Model file for the job. Use its own axes, mm. Face numbers are marked on the shaded views. A direction names the side the tool comes from. Give positions to 0.01 mm unless a question says otherwise; leave off trailing zeros. Loops run counter-clockwise (first coordinate to the right, second up) from the corner with the lowest first, then second, coordinate; pieces in that order, holes last. Notation, with made-up numbers: (-24.5, 34.25) - (-16.5, 34.25) arc R18 ccw to (-16.5, 46.25) - close; hole circle Ø8 at (-15, 10.5). An arc over 180 degrees is marked (long way). Answer as CSV lines item,"result". Start each with the question number.
Item 1: Saw through at C-C on y = 1.75. Give the cut face in (x, z).
Item 2: Drill centre lines: L1, parallel to X at y = 5.5, z = 0; L2, parallel to Y at x = 5, z = 0; L3, parallel to X at y = 1.25, z = 1. Where is each one in solid material? Low to high. Write a range as from..to.
Item 3: Tool access for the marked faces 4 and 5: list every direction of +Z, -Z, +X, -X, +Y, -Y with a clear straight run to the whole face (end or side of a thin tool).
Item 4: Pull direction X, two halves, no side cores. Call the marked faces 1, 2 and 3: pulls with the +X half, pulls with the -X half, needs draft (parallel to the pull), parting line crosses it, or undercut.
Item 5: Pin check, flat tips, straight feed: pin 1 (3 mm diameter, centred on x = 0.5, y = 7, fed in from -Z); pin 2 (1 mm diameter, centred on x = -1.5, y = 3, fed in from +Z); pin 3 (2 mm diameter, centred on x = -1.5, y = 0.5, fed in from +Z). Stop position of each tip, or through.
from build123d import *

# Parameters (mm, degrees)
SKETCH_1_R           = 6
SKETCH_1_R_2         = 1.5
EXTRUDE_1_DEPTH      = 0.9
EXTRUDE_2_DEPTH      = 7.3
EXTRUDE_2_DEPTH_BACK = 1.3
SKETCH_2_R           = 2.45
SKETCH_2_R_2         = 1.5
SKETCH_3_OUTSIDE_W   = 17.806
SKETCH_3_OUTSIDE_H   = 17.806
SKETCH_3_OUTSIDE_R   = 2.425
SKETCH_3_OUTSIDE_R_2 = 1.5
CUT_EXTRUDE_1_DEPTH  = 2
FILLET_1_R           = 0.1
FILLET_2_R           = 0.1
CHAMFER_1_SIZE       = 0.4
CHAMFER_1_SIZE2      = 1


with BuildPart() as part:
    # 草图1 → 凸台-拉伸1 (new body)
    with BuildSketch(Plane(origin=(0, 0, 0), x_dir=(1, 0, 0), z_dir=(0, 1, 0))):
        with Locations(Location((0, 0, 0), (0, 0, 270))):
            Circle(SKETCH_1_R)
        with Locations(Location((0, 0, 0), (0, 0, 270))):
            Circle(SKETCH_1_R_2, mode=Mode.SUBTRACT)
    extrude(amount=EXTRUDE_1_DEPTH)

    # 草图2 → 凸台-拉伸2 (add, two sides: drawn at the far end of the back side and taken through both)
    with BuildSketch(Plane(origin=(0, 0.9, 0), x_dir=(1, 0, 0), z_dir=(0, 1, 0)).offset(-EXTRUDE_2_DEPTH_BACK)):
        with Locations(Location((0, 0, 0), (0, 0, 270))):
            Circle(SKETCH_2_R)
        with Locations(Location((0, 0, 0), (0, 0, 270))):
            Circle(SKETCH_2_R_2, mode=Mode.SUBTRACT)
    extrude(amount=EXTRUDE_2_DEPTH + EXTRUDE_2_DEPTH_BACK)

    # 草图3 outside → 切除-拉伸1 (cut)
    # profile 1 of 2: a face of its own
    with BuildSketch(Plane(origin=(0, 8.2, 0), x_dir=(1, 0, 0), z_dir=(0, 1, 0))):
        Rectangle(SKETCH_3_OUTSIDE_W, SKETCH_3_OUTSIDE_H)
        with Locations(Location((0, 0, 0), (0, 0, 270))):
            Circle(SKETCH_3_OUTSIDE_R, mode=Mode.SUBTRACT)
    # profile 2 of 2: a face of its own
    with BuildSketch(Plane(origin=(0, 8.2, 0), x_dir=(1, 0, 0), z_dir=(0, 1, 0))):
        with Locations(Location((0, 0, 0), (0, 0, 270))):
            Circle(SKETCH_3_OUTSIDE_R_2)
    extrude(amount=-CUT_EXTRUDE_1_DEPTH, mode=Mode.SUBTRACT)

    # 圆角1
    fillet_1_edges = [part.edges().sort_by_distance(p)[0] for p in [
        (0, -0.4, -2.45),
        (0, -0.4, -1.5),
        (0, 8.2, -1.5),
        (0, 8.2, -2.425),
    ]]
    fillet(fillet_1_edges, radius=FILLET_1_R)

    # 圆角2
    # the kernel refuses this fillet: 0.1 mm, written as the material it takes off along each edge
    with BuildSketch(Plane(origin=(0, 6.2, 0), x_dir=(0, 0, 1), z_dir=(1, 0, 0))) as fillet_2_piece_1:
        with BuildLine():
            CenterArc((2.35, 0.066143783), FILLET_2_R, 318.590377891, 41.409622109)
            Line((2.425, 0), (2.4265, -0.001322876))
            ThreePointArc((2.4265, -0.001322876), (2.4375, -0.002), (2.45, -0.002))
            Line((2.45, -0.002), (2.452, 0))
            Line((2.452, 0), (2.452, 0.066143783))
            Line((2.452, 0.066143783), (2.45, 0.066143783))
        make_face()
    revolve(axis=Axis((0, 6.2, 0), (0, -1, 0)), mode=Mode.SUBTRACT)

    # 倒角1
    chamfer_1_edges = [part.edges().sort_by_distance(p)[0] for p in [
        (0, 0.9, -6),
    ]]
    chamfer_1_side = [part.faces().sort_by_distance(p)[0] for p in [
        (0, 0.45, -6),
    ]]
    chamfer(chamfer_1_edges, length=CHAMFER_1_SIZE, length2=CHAMFER_1_SIZE2, reference=chamfer_1_side[0])


solid = part.part
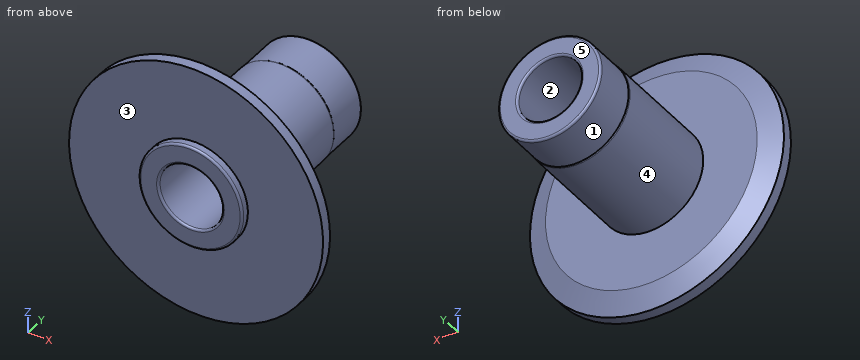
Responses:
1,outline,"circle Ø4.9 at (0, 0); hole circle Ø3 at (0, 0)"
2,L1,"-2.45..-1.5, 1.5..2.45"
2,L2,"0..0.9"
2,L3,"-2.24..-1.12, 1.12..2.24"
3,face 4,"+Y"
3,face 5,"+Z, -Z, +X, -X, +Y"
4,face 1,"parting line crosses it"
4,face 2,"undercut"
4,face 3,"needs draft"
5,pin 1,"z = -2.45"
5,pin 2,"z = 2.24"
5,pin 3,"z = 5.98"
